Design review of the part built by this model. Coordinates are the model's own, in mm. A direction names the side the tool comes from. Coordinates: 2 decimals unless noted, no trailing zeros. Write each loop counter-clockwise with the first axis right and the second up, starting at its lowest first coordinate (ties: lowest second). Pieces come first, ordered by that corner, then holes.
Q1. The part is to be moulded in two halves that separate along X. For faces 4 (the cylindrical face through (2.432, 2.066, 5.866)), 5 (the cylindrical face through (-1.12, -1.79, -0.15)), 6 (the flat face through (-4, 4.191, 0)), 7 (the flat face through (1.5, 2.7, -0.1)), say which applies: released by +X, released by -X, zero draft, split by the parting line, or undercut.
Q2. Take a section at C-C, the plane z = 5.25. Write out the cut boundary in (x, y), plus the area to 3 significant figures.
Q3. For faces 1 (the flat face through (1.2, -6.35, 1.2)), 2 (the cylindrical face through (1.93, -3.43, -2.52)), 3 (the flat face through (-1.5, 2.7, 0.1)), list the 3-axis set-ups (+Z, -Z, +X, -X, +Y, -Y) from which the entire face can be reached by the end or side of a thin tool; tool diameter is ignored.
Q4. Take a section at D-D, the plane x = -5. Write out the cut boundary in (y, z).
Q5. For L1, parallel to X at y = -2.25, z = 0 (3 decimals); L2, parallel to X at y = 0.25, z = 0; L3, parallel to Z at x = 5, y = 2, list the stretches that pass through material, from the lowest coordinate up.
Q6. Take a section at A-A, the plane z = 0. Write out the cut boundary in (x, y) (3 decimals), plus the area to 3 significant figures.
Q7. For pin 1 Ø5 at (y, z) = (-5, 3.5) entering from +X; pin 2 Ø1 at (x, y) = (-2, -1) entering from -Z; pin 3 Ø4 at (y, z) = (-3, -3.5) entering from -X, all flat-tipped, find the tip position at first contact; note any pin that passes through.
Q8. Take a section at B-B, the plane y = 0.5. Write out the cut boundary in (x, z).
from build123d import *

# Parameters (mm, degrees)
CUT_EXTRUDE1_DEPTH      = 7.35
CUT_EXTRUDE1_DEPTH_BACK = 7.35
SKETCH7_W               = 1.1303
SKETCH7_H               = 10.541
CHAMFER1_SIZE           = 0.2921


with BuildPart() as part:
    # Sketch9 → Revolve1 (revolve)
    with BuildSketch(Plane.XY, mode=Mode.PRIVATE) as revolve1_sk:
        Polygon((0, 4.191), (6.35, 4.191), (6.35, 0), (3.175, 0), (3.175, -6.35), (0, -6.35), align=None)
    revolve(revolve1_sk.sketch.rotate(Axis((0, 6.439023264, 0), (0, -1, 0)), 90), axis=Axis((0, 6.439023264, 0), (0, -1, 0)))  # turned: the seam where the file's is

    # Sketch3 → Cut-Extrude1 (cut, two sides)
    with BuildSketch(Plane.XY) as cut_extrude1_sk:
        Polygon((-2.991528061, 4.191), (2.991528061, 4.191), (0, 1.199471939), align=None)
    extrude(amount=CUT_EXTRUDE1_DEPTH, mode=Mode.SUBTRACT)
    extrude(cut_extrude1_sk.sketch, amount=-CUT_EXTRUDE1_DEPTH_BACK, mode=Mode.SUBTRACT)

    # Sketch7 → Cut-Revolve1 (revolve, cut)
    with BuildSketch(Plane.XY, mode=Mode.PRIVATE) as cut_revolve1_sk:
        with Locations((0.56515, -1.0795)):
            Rectangle(SKETCH7_W, SKETCH7_H)
    revolve(cut_revolve1_sk.sketch.rotate(Axis((0, 13.979393491, 0), (0, -1, 0)), 90), axis=Axis((0, 13.979393491, 0), (0, -1, 0)), mode=Mode.SUBTRACT)  # turned: the seam where the file's is

    # Chamfer1
    chamfer1_edges = [part.edges().sort_by_distance(p)[0] for p in [
        (0, -6.35, -1.1303),
        (0, -6.35, -3.175),
    ]]
    chamfer(chamfer1_edges, length=CHAMFER1_SIZE)

    # Sketch10 → Cut-Revolve2 (revolve, cut)
    with BuildSketch(Plane.XY, mode=Mode.PRIVATE) as cut_revolve2_sk:
        with BuildLine():
            Line((3.175, -0.735852294), (3.910852294, 0))
            ThreePointArc((3.910852294, 0), (3.175, 0), (3.175, -0.735852294))
        make_face()
    revolve(cut_revolve2_sk.sketch.rotate(Axis((0, 0, 0), (0, 1, 0)), 270), axis=Axis((0, 0, 0), (0, 1, 0)), mode=Mode.SUBTRACT)  # turned: the seam where the file's is


solid = part.part
Responses:
1. face 4: split by the parting line
1. face 5: undercut
1. face 6: zero draft
1. face 7: undercut
2. outline: (-3.57, 0) - (3.57, 0) - (3.57, 4.19) - (2.99, 4.19) - (0, 1.2) - (-2.99, 4.19) - (-3.57, 4.19) - close
2. area: 21.0 mm2
3. face 1: +Z, -Z, +X, -X, -Y
3. face 2: -Y
3. face 3: +Z, -Z, +Y
4. outline: (0, -3.91) - (4.19, -3.91) - (4.19, 3.91) - (0, 3.91) - close
5. L1: x = -3.175 to -1.13, 1.13 to 3.175
5. L2: x = -6.35 to -1.13, 1.13 to 6.35
5. L3: z = -3.91 to 3.91
6. outline: (-6.35, 0) - (-3.911, 0) arc R0.52 cw to (-3.175, -0.736) - (-3.175, -6.058) - (-2.883, -6.35) - (-1.422, -6.35) - (-1.13, -6.058) - (-1.13, 2.33) - (-2.992, 4.191) - (-6.35, 4.191) - close; (1.13, -6.058) - (1.422, -6.35) - (2.883, -6.35) - (3.175, -6.058) - (3.175, -0.736) arc R0.52 cw to (3.911, 0) - (6.35, 0) - (6.35, 4.191) - (2.992, 4.191) - (1.13, 2.33) - close
6. area: 65.8 mm2
7. pin 1: stops at x = 3.01
7. pin 2: stops at z = -2.8
7. pin 3: stops at x = -2.8
8. outline: circle Ø12.7 at (0, 0); hole circle Ø2.26 at (0, 0)
